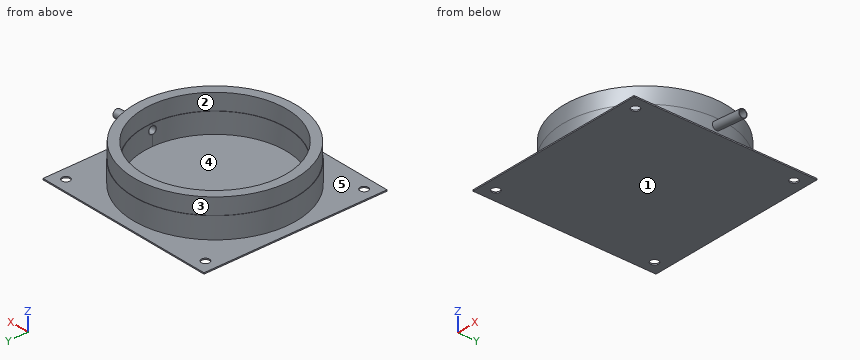
from build123d import *
from build123d import SkipClean  # not in build123d's __all__

# Parameters (mm, degrees)
F0_W     = 10
F0_H     = 3
F2_W     = 450
F2_H     = 450
F2_R     = 10
F3_DEPTH = 3
F6_R     = 9
F7_DEPTH = 120
F8_R     = 175
F9_DEPTH = 200


with BuildPart() as f1:
    # F0 (on Front) → F1 (revolve)
    with BuildSketch(Plane.XZ):
        Polygon((-200, 5), (-175, 5), (-175, 55), (-176, 55), (-176, 95), (-199, 95), (-199, 55), (-200, 55), align=None)
        Polygon((-10, 5), (-175, 5), (-200, 5), (-200, 2), (-10, 2), align=None)
        with Locations((-5, 3.5)):
            Rectangle(F0_W, F0_H)
    revolve(axis=Axis((0, 0, 187.9212413023), (0, 0, -1)))

    # F2 (on Top) → F3 (join)
    with BuildSketch(Plane.XY):
        Rectangle(F2_W, F2_H)
        with Locations((-195, -195)):
            Circle(F2_R, mode=Mode.SUBTRACT)
        with Locations((195, -195)):
            Circle(F2_R, mode=Mode.SUBTRACT)
        with Locations((-195, 195)):
            Circle(F2_R, mode=Mode.SUBTRACT)
        with Locations((195, 195)):
            Circle(F2_R, mode=Mode.SUBTRACT)
    extrude(amount=F3_DEPTH)

    # F4 (on Front) → F5 (revolve)
    with BuildSketch(Plane.XZ):
        Polygon((274.6194698092, 41.5098406888), (175, 50.2254149636), (174.9128442573, 49.2292202655), (274.5323140664, 40.5136459907), align=None)
    revolve(axis=Axis((287.7442754949, 0, 30.3233706049), (0.9961946981, 0, -0.0871557427)))

    # F6 (on face) → F7 (cut)
    with BuildSketch(Plane(origin=(268.9293723072, 0, -23.528271366), x_dir=(0, 1, 0), z_dir=(0.9961946981, 0, -0.0871557427))):
        with Locations((0, 55.286547077)):
            Circle(F6_R)
    extrude(amount=-F7_DEPTH, mode=Mode.SUBTRACT)

    # F8 (on face) → F9 (cut)
    with BuildSketch(Plane.XY.offset(5)):
        Circle(F8_R)
    with SkipClean():  # cleaning this boolean's faces spoils the solid; the shape is the same uncleaned
        extrude(amount=F9_DEPTH, mode=Mode.SUBTRACT)


solid = f1.part
Could you check a few things on this model? Use its own coordinates, in mm. Face numbers are marked on the shaded views. A direction names the side the tool comes from. Coordinates: 2 decimals unless noted, no trailing zeros. Write each loop counter-clockwise with the first axis right and the second up, starting at its lowest first coordinate (ties: lowest second). Pieces come first, ordered by that corner, then holes. Notation, with made-up numbers: (-29.5, 78) - (-8.5, 78) arc R17 cw to (-8.5, 100) - close; hole circle Ø1 at (72.25, -28). An arc over 180 degrees is marked (long way). Write item = value, one per line.
1) Please list where these lines run through material, in increasing order: line 1 (Y direction, x = -195, z = 1.55); line 2 (Y direction, x = 0, z = 86); line 3 (Z direction, x = 70.5, y = -151.5). Write a range as [from, to].
Result set:
line_1 = [-225, -205], [-185, 185], [205, 225]
line_2 = [-199, -176], [176, 199]
line_3 = [0, 5]
2) Suppose I cut it at A-A on x = 0. Please give me the cut outline in (y, z).
Result set:
outline = (-225, 0) - (225, 0) - (225, 3) - (200, 3) - (200, 55) - (199, 55) - (199, 95) - (176, 95) - (176, 55) - (175, 55) - (175, 5) - (-175, 5) - (-175, 55) - (-176, 55) - (-176, 95) - (-199, 95) - (-199, 55) - (-200, 55) - (-200, 3) - (-225, 3) - close
3) Suppose I cut it at B-B on x = 191.5. State how many separate pieces and enclosed holes the cut face has, plus the area to 3 significant figures.
Result set:
separate_pieces = 3
enclosed_holes = 1
area = 11,300 mm2
4) For the marked faces 1 and 2, which set-ups out of +Z, -Z, +X, -X, +Y, -Y let a thin tool reach every point of the face, with its end or its side?
Result set:
face_1 = -Z, +X, -X, +Y, -Y
face_2 = +Z
5) Will these pins go through, and if not, where does the flat tip stop? pin 1 Ø1.5 at (x, z) = (-8.5, 34) entering from +Y; pin 2 Ø5 at (y, z) = (138, 65.5) entering from -X; pin 3 Ø12 at (y, z) = (-140.5, 82.5) entering from -X.
Result set:
pin_1 = 199.85
pin_2 = -145.74
pin_3 = -146.67
6) Suppose I cut it at C-C on y = -162.5. Please give me the cut outline in (x, z).
Result set:
outline = (-225, 0) - (225, 0) - (225, 3) - (116.59, 3) - (116.59, 55) - (114.87, 55) - (114.87, 95) - (67.6, 95) - (67.6, 55) - (64.95, 55) - (64.95, 5) - (-64.95, 5) - (-64.95, 55) - (-67.6, 55) - (-67.6, 95) - (-114.87, 95) - (-114.87, 55) - (-116.59, 55) - (-116.59, 3) - (-225, 3) - close
7) We'd pull the mould along X, two halves only. Please class the marked faces 3, 4 and 5: +X half, -X half, draft (parallel to the pull), parting line (faces both ways), or undercut.
Result set:
face_3 = parting line
face_4 = undercut
face_5 = draft
